from build123d import *
from build123d.topology import SkipClean

# Parameters (mm, degrees)
SKETCH1_W                  = 22
SKETCH1_H                  = 39
SKETCH1_W_2                = 6
SKETCH1_H_2                = 8
BOSS_EXTRUDE1_DEPTH        = 8.25
CUT_EXTRUDE3_DEPTH         = 2.25
SKETCH7_R                  = 2.825
SKETCH7_R_2                = 0.825
CUT_EXTRUDE4_DEPTH         = 1.25
SKETCH9_R                  = 0.75
CUT_EXTRUDE5_DEPTH         = 39.274404999
CUT_EXTRUDE1_DEPTH         = 39.690988331
CUT_EXTRUDE1_DEPTH_BACK    = 39.690988331
SKETCH6_R                  = 2.825
BOSS_EXTRUDE2_DEPTH        = 8.25
FILLET4_R                  = 2
CUT_EXTRUDE7_DEPTH         = 39.900472274
FILLET5_R                  = 7
F_2_2_2_2_DIAMETER_HOLE1_D = 2.2
FILLET6_R                  = 2


with BuildPart() as part:
    # Sketch1 → Boss-Extrude1 (new body)
    with BuildSketch(Plane(origin=(0, 0, 0), x_dir=(1, 0, 0), z_dir=(0, 1, 0))):
        with Locations((21.383330249, 0)):
            Rectangle(SKETCH1_W, SKETCH1_H)
        with Locations((22.383330249, 0)):
            Rectangle(SKETCH1_W_2, SKETCH1_H_2, mode=Mode.SUBTRACT)
    extrude(amount=BOSS_EXTRUDE1_DEPTH)

    # Sketch8 → Cut-Extrude3 (cut)
    with BuildSketch(Plane(origin=(0, 8.25, 0), x_dir=(1, 0, 0), z_dir=(0, 1, 0))):
        Polygon((15.783330249, 17.120672783), (27.383330249, 17.120672783), (30.883330249, 14.183824074), (30.883330249, 8.657521492), (27.383330249, 5.720672783), (15.783330249, 5.720672783), align=None)
        Polygon((27.383330249, -17.120672783), (30.883330249, -14.183824074), (30.883330249, -8.657521492), (27.383330249, -5.720672783), (15.783330249, -5.720672783), (15.783330249, -17.120672783), align=None)
    extrude(amount=-CUT_EXTRUDE3_DEPTH, mode=Mode.SUBTRACT)

    # Sketch7 → Cut-Extrude4 (cut)
    with BuildSketch(Plane(origin=(0, 6, 0), x_dir=(1, 0, 0), z_dir=(0, 1, 0))):
        with Locations(Location((24.633330249, 11.420672783, 0), (0, 0, 270))):
            Circle(SKETCH7_R)
        with Locations(Location((20.140330249, 13.920672783, 0), (0, 0, 270))):
            Circle(SKETCH7_R_2)
        with Locations(Location((27.633330249, 13.920672783, 0), (0, 0, 270))):
            Circle(SKETCH7_R_2)
        with Locations(Location((27.633330249, 8.920672783, 0), (0, 0, 270))):
            Circle(SKETCH7_R_2)
        with Locations(Location((20.140330249, 8.920672783, 0), (0, 0, 270))):
            Circle(SKETCH7_R_2)
        with Locations(Location((20.140330249, -8.920672783, 0), (0, 0, 90))):
            Circle(SKETCH7_R_2)
        with Locations(Location((27.633330249, -8.920672783, 0), (0, 0, 90))):
            Circle(SKETCH7_R_2)
        with Locations(Location((27.633330249, -13.920672783, 0), (0, 0, 90))):
            Circle(SKETCH7_R_2)
        with Locations(Location((20.140330249, -13.920672783, 0), (0, 0, 90))):
            Circle(SKETCH7_R_2)
        with Locations(Location((24.633330249, -11.420672783, 0), (0, 0, 90))):
            Circle(SKETCH7_R)
    extrude(amount=-CUT_EXTRUDE4_DEPTH, mode=Mode.SUBTRACT)

    # Sketch9 → Cut-Extrude5 (cut, through all)
    with BuildSketch(Plane(origin=(0, 6, 0), x_dir=(1, 0, 0), z_dir=(0, 1, 0))):
        with Locations(Location((30.133330249, 11.420672783, 0), (0, 0, 270))):
            Circle(SKETCH9_R)
        with Locations((30.133330249, -11.420672783)):
            Circle(SKETCH9_R)
        with BuildLine():
            Line((16.883330249, 8.920672783), (16.883330249, 13.920672783))
            ThreePointArc((16.883330249, 13.920672783), (17.633330249, 14.670672783), (18.383330249, 13.920672783))
            Line((18.383330249, 13.920672783), (18.383330249, 8.920672783))
            ThreePointArc((18.383330249, 8.920672783), (17.633330249, 8.170672783), (16.883330249, 8.920672783))
        make_face()
        with BuildLine():
            Line((16.883330249, -8.920672783), (16.883330249, -13.920672783))
            ThreePointArc((16.883330249, -13.920672783), (17.633330249, -14.670672783), (18.383330249, -13.920672783))
            Line((18.383330249, -13.920672783), (18.383330249, -8.920672783))
            ThreePointArc((18.383330249, -8.920672783), (17.633330249, -8.170672783), (16.883330249, -8.920672783))
        make_face()
    extrude(amount=-CUT_EXTRUDE5_DEPTH, mode=Mode.SUBTRACT)

    # Sketch6 → Cut-Extrude1 (cut, two sides: drawn at the far end of the back side and taken through both)
    with BuildSketch(Plane(origin=(0, 8.25, 0), x_dir=(-1, 0, 0), z_dir=(0, -1, 0)).offset(-CUT_EXTRUDE1_DEPTH_BACK)):
        with Locations((-24.633330249, -11.420672783)):
            Circle(SKETCH6_R)
        with Locations((-24.633330249, 11.420672783)):
            Circle(SKETCH6_R)
        Polygon((-26.045830249, -8.974151017), (-25.695830249, -9.5803688), (-12.705449192, -2.0803688), (-13.055449192, -1.474151017), align=None)
        Polygon((-13.055449192, 1.474151017), (-12.705449192, 2.0803688), (-25.695830249, 9.5803688), (-26.045830249, 8.974151017), align=None)
    extrude(amount=CUT_EXTRUDE1_DEPTH + CUT_EXTRUDE1_DEPTH_BACK, mode=Mode.SUBTRACT)

    # Sketch11 → Boss-Extrude2 (add, through all)
    with BuildSketch(Plane(origin=(0, 8.25, 0), x_dir=(1, 0, 0), z_dir=(0, 1, 0))):
        with BuildLine():
            ThreePointArc((32.383330249, 10.221714902), (32.633330249, 11.420672783), (32.383330249, 12.619630664))
            Line((32.383330249, 12.619630664), (32.383330249, 10.221714902))
        make_face()
        with BuildLine():
            ThreePointArc((32.383330249, -12.619630664), (32.633330249, -11.420672783), (32.383330249, -10.221714902))
            Line((32.383330249, -10.221714902), (32.383330249, -12.619630664))
        make_face()
    extrude(amount=-BOSS_EXTRUDE2_DEPTH)

    # Fillet4
    fillet4_edges = [part.edges().sort_by_distance(p)[0] for p in [
        (25.383330249, 4.125, -4),
        (19.383330249, 4.125, -4),
        (19.383330249, 4.125, 4),
        (25.383330249, 4.125, 4),
    ]]
    fillet(fillet4_edges, radius=FILLET4_R)

    # Sketch11<4> → Cut-Extrude7 (cut, through all)
    with SkipClean():  # the faces are left unmerged after this step: merging them gives an invalid solid
        with BuildSketch(Plane(origin=(0, 8.25, 0), x_dir=(1, 0, 0), z_dir=(0, 1, 0))):
            with BuildLine():
                Line((29.633330249, 17.420672783), (32.231406461, 12.920672783))
                ThreePointArc((32.231406461, 12.920672783), (32.311601404, 12.772287972), (32.383330249, 12.619630664))
                Line((32.383330249, 12.619630664), (32.383330249, 19.5))
                Line((32.383330249, 19.5), (28.432830121, 19.5))
                Line((28.432830121, 19.5), (29.633330249, 17.420672783))
            make_face()
            with BuildLine():
                Line((32.383330249, -10.221714902), (32.383330249, 10.221714902))
                ThreePointArc((32.383330249, 10.221714902), (32.311601404, 10.069057593), (32.231406461, 9.920672783))
                Line((32.231406461, 9.920672783), (29.633330249, 5.420672783))
                Line((29.633330249, 5.420672783), (29.633330249, -5.420672783))
                Line((29.633330249, -5.420672783), (32.231406461, -9.920672783))
                ThreePointArc((32.231406461, -9.920672783), (32.311601404, -10.069057593), (32.383330249, -10.221714902))
            make_face()
            with BuildLine():
                Line((32.383330249, -19.5), (32.383330249, -12.619630664))
                ThreePointArc((32.383330249, -12.619630664), (32.311601404, -12.772287972), (32.231406461, -12.920672783))
                Line((32.231406461, -12.920672783), (29.633330249, -17.420672783))
                Line((29.633330249, -17.420672783), (28.432830121, -19.5))
                Line((28.432830121, -19.5), (32.383330249, -19.5))
            make_face()
        extrude(amount=-CUT_EXTRUDE7_DEPTH, mode=Mode.SUBTRACT)

    # Fillet5
    fillet5_edges = [part.edges().sort_by_distance(p)[0] for p in [
        (10.383330249, 4.125, 19.5),
        (10.383330249, 4.125, -19.5),
    ]]
    fillet(fillet5_edges, radius=FILLET5_R)

    # Ø2.2 (2.2) Diameter Hole1 (through all)
    with Locations(Plane(origin=(12.883330249, 8.25, -12), x_dir=(0, 0, 1), z_dir=(0, 1, 0))):
        with Locations((0, 0), (12, 14.5), (24, 0)):
            Hole(F_2_2_2_2_DIAMETER_HOLE1_D / 2)

    # Fillet6
    fillet6_edges = [part.edges().sort_by_distance(p)[0] for p in [
        (28.432830121, 4.125, -19.5),
        (28.432830121, 4.125, 19.5),
    ]]
    fillet(fillet6_edges, radius=FILLET6_R)


solid = part.part
Here's how the part is built. I have some questions about the finished solid (model axes, mm). A direction names the side the tool comes from. Round coordinates to 2 decimals unless told otherwise and drop trailing zeros. Write each loop counter-clockwise with the first axis right and the second up, starting at its lowest first coordinate (ties: lowest second). Pieces come first, ordered by that corner, then holes.
1. Will these pins go through, and if not, where does the flat tip stop? pin 1 Ø3 at (x, y) = (15, 6.5) entering from +Z; pin 2 Ø1.5 at (y, z) = (7, -3) entering from +X; pin 3 Ø0.5 at (x, z) = (27.5, -8.5) entering from +Y.
2. If we mould it in two halves opening along X, with no side actions, what happens to faces 3 (the cylindrical face through (26.83, 5.38, -14.1)), 4 (the flat face through (22, 7, -17.121)), 5 (the cylindrical face through (12.379, 4.183, -17.395))? For each: released by +X, released by -X, zero draft, split by the parting line, or undercut.
3. Suppose I cut it at B-B (y = 1.5). State how many separate pieces and enclosed holes the cut face has, and give its area (3 significant figures).
4. For faces 1 (the flat face through (18.383, 3, -11)), 2 (the flat face through (20, 4.75, -14)), which set-ups out of +Z, -Z, +X, -X, +Y, -Y let a thin tool reach every point of the face, with its end or its side?
5. Suppose I cut it at A-A (z = 0). List the corners of the cut face in (x, y) for me.
6. I need wall thicknesses on L1, parallel to Z at x = 21.25, y = 6.75; L2, parallel to Z at x = 23.25, y = 5.75; L3, parallel to X at y = 7.75, z = 11.5. Which ranges of each line are inside material? Lowest first, please.
Answer sheet:
1. pin 1: stops at z = 19.44
1. pin 2: stops at x = 29.63
1. pin 3: stops at y = 4.75
2. face 3: undercut
2. face 4: undercut
2. face 5: released by -X
3. separate pieces: 1
3. enclosed holes: 10
3. area: 620 mm2
4. face 1: +Y, -Y
4. face 2: +Y
5. outline: (10.38, 0) - (19.38, 0) - (19.38, 8.25) - (10.38, 8.25) - close; (25.38, 0) - (26.28, 0) - (26.28, 8.25) - (25.38, 8.25) - close; (28.48, 0) - (29.63, 0) - (29.63, 8.25) - (28.48, 8.25) - close
6. L1: z = -19.5 to -17.12, -5.72 to -4, 4 to 5.72, 17.12 to 19.5
6. L2: z = -19.5 to -13.88, -8.96 to -8.17, -7.36 to -4, 4 to 7.36, 8.17 to 8.96, 13.88 to 19.5
6. L3: x = 10.38 to 11.9, 13.86 to 15.78, 30.88 to 32.63
